Autodesk Inventor part; units mm, degrees
ref_plane "YZ Plane" through (0, 0, 0) normal (1, 0, 0) x (0, 1, 0)
ref_plane "XZ Plane" through (0, 0, 0) normal (0, 1, 0) x (-1, 0, 0)
ref_plane "XY Plane" through (0, 0, 0) normal (0, 0, 1) x (1, 0, 0)
sketch "Sketch1" plane through (0, 0, 0) normal (0, 0, 1) x (1, 0, 0)
  circle A0 centre (0, 0) radius 3.5
  dimension "d0" = 7
extrude "Extrusion1" add sketch "Sketch1" along normal mid plane 100
sketch "Sketch2" plane through (0, 0, 0) normal (0, 1, 0) x (-1, 0, 0)
  circle A0 centre (0, 45) radius 2.5
  circle A1 centre (0, -45) radius 2.5
  point P0 (0, 0)
  dimension "d3" = 5
  dimension "d4" = 45
  dimension "d5" = 5
  dimension "d6" = 45
extrude "Extrusion2" cut sketch "Sketch2" along normal through all both and the other way through all
thread "Thread1"
thread "Thread2"
Model file for the job. Use its own axes, mm. Coordinates: 2 decimals unless noted, no trailing zeros. Write each loop counter-clockwise with the first axis right and the second up, starting at its lowest first coordinate (ties: lowest second). Pieces come first, ordered by that corner, then holes. Notation, with made-up numbers: (71.5, 29) - (123.5, 29) arc R29 ccw to (123.5, 61) - close; hole circle Ø5 at (-38, 85). An arc over 180 degrees is marked (long way). Write each question's results on one line, items separated by ' | '. Start each with the question number.
1) Cut at B-B (y = 0). Write the cut outline in (x, z).
2) Probe line 1 along Z through (x, y) = (0, 0.5); line 2 along Z through (x, y) = (0.5, 0.75); line 3 along X through (y, z) = (-0.25, -21.5). List the from-to ranges inside material, lowest first. Write a range as from..to.
3) Cut at A-A (x = 0). Write the cut outline in (y, z).
4) Flat gauge pins, fed straight in: P1, Ø3, axis at x = 2.5, z = -17, coming from the +Y side; P2, Ø1.5, axis at x = 2.5, z = 5.5, coming from the +Y side. Where does each tip first touch, or does it go through?
5) Cut at C-C (z = 30). Write the cut outline in (x, y).
6) Cut at D-D (z = -45). Write the cut outline in (x, y), then the cut area to 3 significant figures.
Returned:
1) outline: (-3.5, -50) - (3.5, -50) - (3.5, 50) - (-3.5, 50) - close; hole circle Ø5 at (0, -45); hole circle Ø5 at (0, 45)
2) line 1: -50..-47.5, -42.5..42.5, 47.5..50 | line 2: -50..-47.45, -42.55..42.55, 47.45..50 | line 3: -3.49..3.49
3) outline: (-3.5, -50) - (3.5, -50) - (3.5, -47.5) - (-3.5, -47.5) - close; (-3.5, -42.5) - (3.5, -42.5) - (3.5, 42.5) - (-3.5, 42.5) - close; (-3.5, 47.5) - (3.5, 47.5) - (3.5, 50) - (-3.5, 50) - close
4) P1: y = 3.35 | P2: y = 3.03
5) outline: circle Ø7 at (0, 0)
6) outline: (-2.5, -2.45) - (-2.5, 2.45) arc R3.5 ccw to start; (2.5, -2.45) arc R3.5 ccw to (2.5, 2.45) - close | area: 6.74 mm^2
